from build123d import *

# Parameters (mm, degrees)
AUFSATZ_LINEAR_AUSTRAGEN1_DEPTH  = 40
SCHNITT_LINEAR_AUSTRAGEN3_DEPTH  = 40
SCHNITT_LINEAR_START             = -6
SCHNITT_LINEAR_AUSTRAGEN4_DEPTH  = 6
SCHNITT_LINEAR_AUSTRAGEN5_DEPTH  = 6
VERRUNDUNG1_R                    = 3
SCHNITT_LINEAR_AUSTRAGEN6_REACH  = 45.817
SKIZZE5_R                        = 1.7
SCHNITT_LINEAR_AUSTRAGEN7_REACH  = 49.001
SKIZZE6_R                        = 1.7
SCHNITT_ROTATION_D_NN1_START     = 26.307192439
SCHNITT_ROTATION_D_NN1_OUTLINE_R = 1.5
SCHNITT_ROTATION_D_NN1_DEPTH     = 11.713572656
SCHNITT_ROTATION_D_NN2_START     = -1.977078808
SCHNITT_ROTATION_D_NN2_OUTLINE_R = 1.5
SCHNITT_ROTATION_D_NN2_DEPTH     = 11.713571611
VERRUNDUNG2_R                    = 1
SCHNITT_LINEAR_AUSTRAGEN8_DEPTH  = 2
SCHNITT_LINEAR_AUSTRAGEN9_REACH  = 45.817
SKIZZE10_R                       = 2.3
SKIZZE10_R_2                     = 1.7


# Read off the part's stored shape, not the designer's step: Schnitt-Rotation-Dünn1, Schnitt-Rotation-Dünn2
with BuildPart() as part:
    # Skizze1 → Aufsatz-Linear austragen1 (new body)
    with BuildSketch(Plane(origin=(0, 0, 0), x_dir=(1, 0, 0), z_dir=(0, 1, 0))):
        with BuildLine():
            Line((-5.759831503, 14.966295554), (13.068371728, 14.966295554))
            ThreePointArc((13.068371728, 14.966295554), (14.621285998, 14.761850511), (16.068371728, 14.162447976))
            Line((16.068371728, 14.162447976), (24.666447939, 9.198346361))
            Line((24.666447939, 9.198346361), (22.166447939, 4.868219342))
            Line((22.166447939, 4.868219342), (14.728625766, 9.162447976))
            ThreePointArc((14.728625766, 9.162447976), (13.281540036, 9.761850511), (11.728625766, 9.966295554))
            Line((11.728625766, 9.966295554), (-5.759831503, 9.966295554))
            Line((-5.759831503, 9.966295554), (-5.759831503, 14.966295554))
        make_face()
    extrude(amount=AUFSATZ_LINEAR_AUSTRAGEN1_DEPTH)

    # Skizze2 → Schnitt-Linear austragen3 (cut)
    with BuildSketch(Plane(origin=(0, 40, 0), x_dir=(1, 0, 0), z_dir=(0, 1, 0))):
        Polygon((-5.759831503, 14.966295554), (-5.759831503, 12.966295554), (-2.295729887, 14.966295554), align=None)
        Polygon((24.666447939, 9.198346361), (22.934397132, 10.198346361), (23.666447939, 7.466295554), align=None)
    extrude(amount=-SCHNITT_LINEAR_AUSTRAGEN3_DEPTH, mode=Mode.SUBTRACT)

    # Skizze3 → Schnitt-Linear austragen4 (cut)
    with BuildSketch(Plane(origin=(0, 40, 0), x_dir=(1, 0, 0), z_dir=(0, 1, 0)).offset(SCHNITT_LINEAR_START)):
        with BuildLine():
            Line((-5.759831503, 12.966295554), (12.532473343, 12.966295554))
            ThreePointArc((12.532473343, 12.966295554), (14.085387613, 12.761850511), (15.532473343, 12.162447976))
            Line((15.532473343, 12.162447976), (21.181781368, 8.900818467))
            ThreePointArc((21.181781368, 8.900818467), (23.993765179, 5.194915748), (23.31194468, 0.593167307))
            Line((23.31194468, 0.593167307), (22.166447939, 4.868219342))
            Line((22.166447939, 4.868219342), (14.728625766, 9.162447976))
            ThreePointArc((14.728625766, 9.162447976), (13.281540036, 9.761850511), (11.728625766, 9.966295554))
            Line((11.728625766, 9.966295554), (-5.759831503, 9.966295554))
            Line((-5.759831503, 9.966295554), (-5.759831503, 12.966295554))
        make_face()
    extrude(amount=SCHNITT_LINEAR_AUSTRAGEN4_DEPTH, mode=Mode.SUBTRACT)

    # Skizze4 → Schnitt-Linear austragen5 (cut)
    with BuildSketch(Plane.XZ):
        with BuildLine():
            Line((21.181781368, -8.900818467), (15.532473343, -12.162447976))
            ThreePointArc((15.532473343, -12.162447976), (14.085387614, -12.761850511), (12.532473343, -12.966295554))
            Line((12.532473343, -12.966295554), (-5.759831503, -12.966295554))
            Line((-5.759831503, -12.966295554), (-5.759831503, -9.966295554))
            Line((-5.759831503, -9.966295554), (11.728625766, -9.966295554))
            ThreePointArc((11.728625766, -9.966295554), (13.281540036, -9.761850511), (14.728625766, -9.162447976))
            Line((14.728625766, -9.162447976), (22.166447939, -4.868219342))
            Line((22.166447939, -4.868219342), (23.31194468, -0.593167307))
            ThreePointArc((23.31194468, -0.593167307), (23.993765179, -5.194915748), (21.181781368, -8.900818467))
        make_face()
    extrude(amount=-SCHNITT_LINEAR_AUSTRAGEN5_DEPTH, mode=Mode.SUBTRACT)

    # Verrundung1
    verrundung1_edges = [part.edges().sort_by_distance(p)[0] for p in [
        (22.934397132, 20, -10.198346361),
        (-2.295729887, 20, -14.966295554),
        (22.166447939, 20, -4.868219342),
        (-5.759831503, 20, -9.966295554),
    ]]
    fillet(verrundung1_edges, radius=VERRUNDUNG1_R - 0.0001)  # a hair under: the kernel refuses the full size

    # Skizze5 → Schnitt-Linear austragen6 (cut, up to next)
    with BuildSketch(Plane(origin=(9.149612796, 0, -15.847594231), x_dir=(0.8660254037844386, 0, 0.5000000000000003), z_dir=(-0.5000000000000002, 0, 0.8660254037844385)), mode=Mode.PRIVATE) as schnitt_linear_austragen6_sk1:
        with Locations((10.37029251, 3)):
            Circle(SKIZZE5_R)
    schnitt_linear_austragen6_tool1 = extrude(schnitt_linear_austragen6_sk1.sketch, amount=-SCHNITT_LINEAR_AUSTRAGEN6_REACH, mode=Mode.PRIVATE) & part.part
    # Skizze5 → Schnitt-Linear austragen6 (cut, up to next)
    with BuildSketch(Plane(origin=(9.149612796, 0, -15.847594231), x_dir=(0.8660254037844386, 0, 0.5000000000000003), z_dir=(-0.5000000000000002, 0, 0.8660254037844385)), mode=Mode.PRIVATE) as schnitt_linear_austragen6_sk2:
        with Locations((10.37029251, 37)):
            Circle(SKIZZE5_R)
    schnitt_linear_austragen6_tool2 = extrude(schnitt_linear_austragen6_sk2.sketch, amount=-SCHNITT_LINEAR_AUSTRAGEN6_REACH, mode=Mode.PRIVATE) & part.part
    add(schnitt_linear_austragen6_tool1.solids().sort_by_distance((18.13055, 3, -10.662448))[0], mode=Mode.SUBTRACT)
    add(schnitt_linear_austragen6_tool2.solids().sort_by_distance((18.13055, 37, -10.662448))[0], mode=Mode.SUBTRACT)

    # Skizze6 → Schnitt-Linear austragen7 (cut, up to next)
    with BuildSketch(Plane.XY.offset(-12.966295554), mode=Mode.PRIVATE) as schnitt_linear_austragen7_sk1:
        with Locations((5.532473343, 3)):
            Circle(SKIZZE6_R)
    schnitt_linear_austragen7_tool1 = extrude(schnitt_linear_austragen7_sk1.sketch, amount=-SCHNITT_LINEAR_AUSTRAGEN7_REACH, mode=Mode.PRIVATE) & part.part
    # Skizze6 → Schnitt-Linear austragen7 (cut, up to next)
    with BuildSketch(Plane.XY.offset(-12.966295554), mode=Mode.PRIVATE) as schnitt_linear_austragen7_sk2:
        with Locations((5.532473343, 37)):
            Circle(SKIZZE6_R)
    schnitt_linear_austragen7_tool2 = extrude(schnitt_linear_austragen7_sk2.sketch, amount=-SCHNITT_LINEAR_AUSTRAGEN7_REACH, mode=Mode.PRIVATE) & part.part
    add(schnitt_linear_austragen7_tool1.solids().sort_by_distance((5.532473, 3, -12.966296))[0], mode=Mode.SUBTRACT)
    add(schnitt_linear_austragen7_tool2.solids().sort_by_distance((5.532473, 37, -12.966296))[0], mode=Mode.SUBTRACT)

    # Schnitt-Rotation-Dünn1 outline → Schnitt-Rotation-Dünn1 (cut)
    with BuildSketch(Plane(origin=(0, 0, 0), x_dir=(0.9354143466934868, -0.26726124191241973, 0.23145502494313744), z_dir=(0.35355339059326996, 0.7071067811865439, -0.6123724356958009)).offset(SCHNITT_ROTATION_D_NN1_START)):
        with Locations((1.011284538, -9.386188067)):
            Circle(SCHNITT_ROTATION_D_NN1_OUTLINE_R)
    extrude(amount=SCHNITT_ROTATION_D_NN1_DEPTH, mode=Mode.SUBTRACT)

    # Schnitt-Rotation-Dünn2 outline → Schnitt-Rotation-Dünn2 (cut)
    with BuildSketch(Plane(origin=(0, 0, 0), x_dir=(0.9354143466934868, 0.26726124191241973, 0.23145502494313744), z_dir=(0.35355339059326996, -0.7071067811865439, -0.6123724356958009)).offset(SCHNITT_ROTATION_D_NN2_START)):
        with Locations((11.701734215, -16.799958762)):
            Circle(SCHNITT_ROTATION_D_NN2_OUTLINE_R)
    extrude(amount=SCHNITT_ROTATION_D_NN2_DEPTH, mode=Mode.SUBTRACT)

    # Verrundung2
    verrundung2_edges = [part.edges().sort_by_distance(p)[0] for p in [
        (23.666447939, 20, -7.466295554),
    ]]
    fillet(verrundung2_edges, radius=VERRUNDUNG2_R)

    # Skizze9 → Schnitt-Linear austragen8 (cut)
    with BuildSketch(Plane(origin=(10.149612796, 0, -17.579645039), x_dir=(-0.8660254037844383, 0, -0.5000000000000007), z_dir=(0.5000000000000007, 0, -0.8660254037844383))):
        Polygon((-7.177175397, 26.192388155), (-7.177175397, 13.807611845), (-8.984787242, 12), (-11.369563553, 12), (-13.177175397, 13.807611845), (-13.177175397, 26.192388155), (-11.369563553, 28), (-8.984787242, 28), align=None)
    extrude(amount=-SCHNITT_LINEAR_AUSTRAGEN8_DEPTH, mode=Mode.SUBTRACT)

    # Skizze10 → Schnitt-Linear austragen9 (cut, up to next)
    with BuildSketch(Plane(origin=(9.149612796, 0, -15.847594231), x_dir=(-0.8660254037844384, 0, -0.5000000000000007), z_dir=(0.5000000000000007, 0, -0.8660254037844384)), mode=Mode.PRIVATE) as schnitt_linear_austragen9_sk1:
        with Locations((-10.177175397, 20)):
            Circle(SKIZZE10_R)
    schnitt_linear_austragen9_tool1 = extrude(schnitt_linear_austragen9_sk1.sketch, amount=-SCHNITT_LINEAR_AUSTRAGEN9_REACH, mode=Mode.PRIVATE) & part.part
    # Skizze10 → Schnitt-Linear austragen9 (cut, up to next)
    with BuildSketch(Plane(origin=(9.149612796, 0, -15.847594231), x_dir=(-0.8660254037844384, 0, -0.5000000000000007), z_dir=(0.5000000000000007, 0, -0.8660254037844384)), mode=Mode.PRIVATE) as schnitt_linear_austragen9_sk2:
        with Locations((-10.177175397, 25.8)):
            Circle(SKIZZE10_R_2)
    schnitt_linear_austragen9_tool2 = extrude(schnitt_linear_austragen9_sk2.sketch, amount=-SCHNITT_LINEAR_AUSTRAGEN9_REACH, mode=Mode.PRIVATE) & part.part
    # Skizze10 → Schnitt-Linear austragen9 (cut, up to next)
    with BuildSketch(Plane(origin=(9.149612796, 0, -15.847594231), x_dir=(-0.8660254037844384, 0, -0.5000000000000007), z_dir=(0.5000000000000007, 0, -0.8660254037844384)), mode=Mode.PRIVATE) as schnitt_linear_austragen9_sk3:
        with Locations((-10.177175397, 14.2)):
            Circle(SKIZZE10_R_2)
    schnitt_linear_austragen9_tool3 = extrude(schnitt_linear_austragen9_sk3.sketch, amount=-SCHNITT_LINEAR_AUSTRAGEN9_REACH, mode=Mode.PRIVATE) & part.part
    add(schnitt_linear_austragen9_tool1.solids().sort_by_distance((17.963305, 20, -10.759007))[0], mode=Mode.SUBTRACT)
    add(schnitt_linear_austragen9_tool2.solids().sort_by_distance((17.963305, 25.8, -10.759007))[0], mode=Mode.SUBTRACT)
    add(schnitt_linear_austragen9_tool3.solids().sort_by_distance((17.963305, 14.2, -10.759007))[0], mode=Mode.SUBTRACT)


solid = part.part
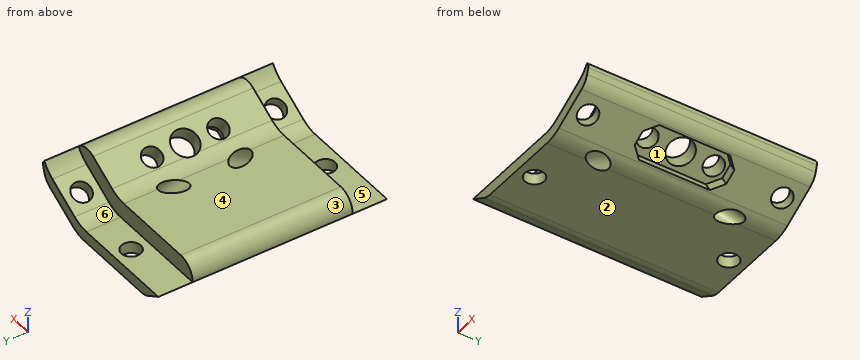
The listing builds one solid part. Answer for the finished solid, in the listing's coordinates (mm). Face numbers are marked on the shaded views. A direction names the side the tool comes from. Give positions to 0.01 mm unless a question says otherwise; leave off trailing zeros. Loops run counter-clockwise (first coordinate to the right, second up) from the corner with the lowest first, then second, coordinate; pieces in that order, holes last. Notation, with made-up numbers: (77.25, -29.75) - (124.25, -29.75) arc R19 cw to (124.25, -8.75) - close; hole circle Ø10 at (63, 70). An arc over 180 degrees is marked (long way). Answer as a JSON object with one key per item and string values.
1. Find the intervals of material crossed by L1, parallel to X at y = 12.5, z = -11; L2, parallel to Y at x = 16.5, z = -10.5; L3, parallel to Y at x = 10.5, z = -10.75, in increasing order. Write a range as [from, to].
Determined:
{"L1": "[-5.03, 10.09], [13.23, 17.55], [20.06, 21.55]", "L2": "[6, 12.94], [15.46, 18], [22, 24.54], [27.06, 34]", "L3": "[6, 11.87], [15.52, 24.48], [28.13, 34]"}
2. A cutting plane is placed at A-A (x = 5.5). Write down the section's boundary in (y, z).
Determined:
{"outline": "(0, -14.97) - (1.3, -14.97) - (1.3, -12.97) - (0, -12.97) - close; (4.7, -14.97) - (35.3, -14.97) - (35.3, -12.97) - (34, -12.97) - (34, -9.97) - (6, -9.97) - (6, -12.97) - (4.7, -12.97) - close; (38.7, -14.97) - (40, -14.97) - (40, -12.97) - (38.7, -12.97) - close"}
3. A cutting plane is placed at B-B (y = 3). Give the number of separate pieces and of enclosed holes in the cut face, then the cut area to 3 significant figures.
Determined:
{"separate pieces": "3", "enclosed holes": "0", "area": "44.2 mm²"}
4. For a pull along X with two mould halves and no side action, classify the marked faces 1, 2 and 3 as pulls with the +X half, pulls with the -X half, needs draft (parallel to the pull), parting line crosses it, or undercut.
Determined:
{"face 1": "undercut", "face 2": "needs draft", "face 3": "pulls with the -X half"}
5. Flat-ended cylindrical pins translate along their axes: pin 1 Ø3 at (x, y) = (-2.5, 8) entering from +Z; pin 2 Ø3 at (x, y) = (7, 3.5) entering from +Z; pin 3 Ø11.5 at (x, y) = (7, 22) entering from +Z; pin 4 Ø2.5 at (x, y) = (5.53, 37) entering from -Z. Find the tip coordinate at first contact, or state that the pin passes through.
Determined:
{"pin 1": "z = -9.97", "pin 2": "z = -12.97", "pin 3": "z = -9.88", "pin 4": "through"}
6. For the marked faces 4, 5 and 6, determine the directions among +Z, -Z, +X, -X, +Y, -Y from which every point of the face is accessible in a straight line to the end or side of a thin tool.
Determined:
{"face 4": "+Z, -X, +Y, -Y", "face 5": "+Z, -X, -Y", "face 6": "+Z, -X, +Y"}
